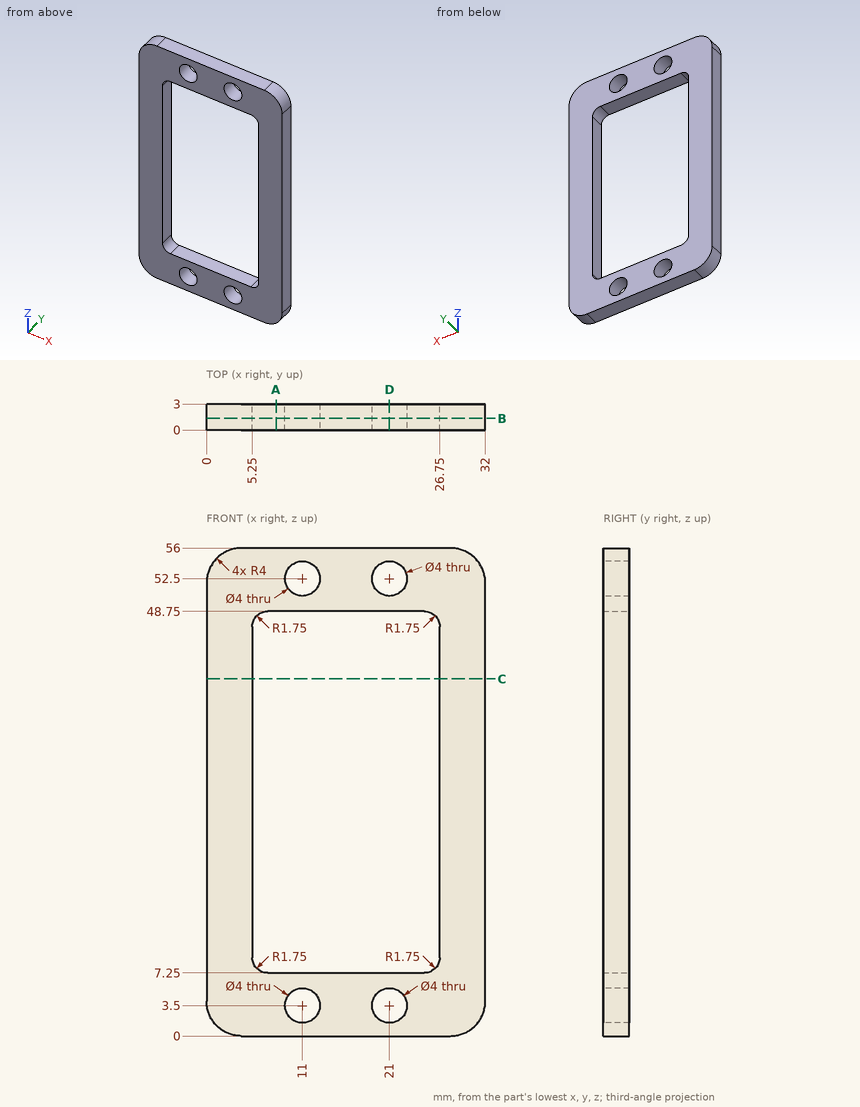
Drawing for the job (mm, zero at the part's lowest x, y, z). Round coordinates to 2 decimals unless told otherwise and drop trailing zeros. Order: outer loops, then holes, each group sorted by start corner. A loop starts at its lowest first (then second) coordinate and runs counter-clockwise, first axis right, second up.
Item 1: Probe line 1 along Z through (x, y) = (21, 1.3); line 2 along X through (y, z) = (0.6, 35); line 3 along Z through (x, y) = (9.5, 1.25). List the from-to ranges inside material, lowest first.
Item 2: Saw through at C-C on z = 41. Write the cut outline in (x, y), then the cut area to 3 significant figures.
Item 3: Saw through at A-A on x = 8. Write the cut outline in (y, z).
Item 4: Saw through at D-D on x = 21. Write the cut outline in (y, z), then the cut area to 3 significant figures.
Item 5: Saw through at B-B on y = 1.35. Write the cut outline in (x, z).
Reported:
1. line 1: z = 0 to 1.5, 5.5 to 7.25, 48.75 to 50.5, 54.5 to 56
1. line 2: x = 0 to 5.25, 26.75 to 32
1. line 3: z = 0 to 2.18, 4.82 to 7.25, 48.75 to 51.18, 53.82 to 56
2. outline: (0, 0) - (5.25, 0) - (5.25, 3) - (0, 3) - close; (26.75, 0) - (32, 0) - (32, 3) - (26.75, 3) - close
2. area: 31.5 mm2
3. outline: (0, 0) - (3, 0) - (3, 7.25) - (0, 7.25) - close; (0, 48.75) - (3, 48.75) - (3, 56) - (0, 56) - close
4. outline: (0, 0) - (3, 0) - (3, 1.5) - (0, 1.5) - close; (0, 5.5) - (3, 5.5) - (3, 7.25) - (0, 7.25) - close; (0, 48.75) - (3, 48.75) - (3, 50.5) - (0, 50.5) - close; (0, 54.5) - (3, 54.5) - (3, 56) - (0, 56) - close
4. area: 19.5 mm2
5. outline: (0, 4) arc R4 ccw to (4, 0) - (28, 0) arc R4 ccw to (32, 4) - (32, 52) arc R4 ccw to (28, 56) - (4, 56) arc R4 ccw to (0, 52) - close; hole (5.25, 9) arc R1.75 ccw to (7, 7.25) - (25, 7.25) arc R1.75 ccw to (26.75, 9) - (26.75, 47) arc R1.75 ccw to (25, 48.75) - (7, 48.75) arc R1.75 ccw to (5.25, 47) - close; hole circle Ø4 at (11, 3.5); hole circle Ø4 at (11, 52.5); hole circle Ø4 at (21, 3.5); hole circle Ø4 at (21, 52.5)
